For this review, take the finished solid that the model builds, in its own axes (mm). Give positions to 0.01 mm unless a question says otherwise; leave off trailing zeros. Loops run counter-clockwise (first coordinate to the right, second up) from the corner with the lowest first, then second, coordinate; pieces in that order, holes last.
```python
from build123d import *

# Parameters (mm, degrees)
F1_DEPTH        = 6
F2_R            = 1
F3_R            = 5
F4_DEPTH        = 1.8
F6_D            = 2.8
F6_CBORE_D      = 6
F6_CBORE_DEPTH  = 2.5
F7_SIZE         = 3
F9_DEPTH        = 0.4
F10_D           = 2.8
F10_CBORE_D     = 6
F10_CBORE_DEPTH = 2.5
F11_R           = 6.1
F12_DEPTH       = 4
F14_DEPTH       = 1


with BuildPart() as f1:
    # F0 (on Right) → F1 (new body)
    with BuildSketch(Plane.YZ):
        Polygon((40.0512183458, -60), (50, -60), (50, 60), (-50, 60), (-50, -60), (-40, -60), (-29.9487816542, -50), (30.0512183458, -50), align=None)
        with BuildLine():
            Line((2.1213203436, -9.1923881554), (32.9289321881, -40))
            Line((32.9289321881, -40), (-32.9289321881, -40))
            Line((-32.9289321881, -40), (-2.1213203436, -9.1923881554))
            ThreePointArc((-2.1213203436, -9.1923881554), (0, -8.313708499), (2.1213203436, -9.1923881554))
        make_face(mode=Mode.SUBTRACT)
        with BuildLine():
            Line((-9.1923881554, -2.1213203436), (-40, -32.9289321881))
            Line((-40, -32.9289321881), (-40, 32.9289321881))
            Line((-40, 32.9289321881), (-9.1923881554, 2.1213203436))
            ThreePointArc((-9.1923881554, 2.1213203436), (-8.313708499, 0), (-9.1923881554, -2.1213203436))
        make_face(mode=Mode.SUBTRACT)
        with BuildLine():
            Line((40, 32.9289321881), (40, -32.9289321881))
            Line((40, -32.9289321881), (9.1923881554, -2.1213203436))
            ThreePointArc((9.1923881554, -2.1213203436), (8.313708499, 0), (9.1923881554, 2.1213203436))
            Line((9.1923881554, 2.1213203436), (40, 32.9289321881))
        make_face(mode=Mode.SUBTRACT)
        with BuildLine():
            Line((-32.9289321881, 40), (32.9289321881, 40))
            Line((32.9289321881, 40), (2.1213203436, 9.1923881554))
            ThreePointArc((2.1213203436, 9.1923881554), (0, 8.313708499), (-2.1213203436, 9.1923881554))
            Line((-2.1213203436, 9.1923881554), (-32.9289321881, 40))
        make_face(mode=Mode.SUBTRACT)
    extrude(amount=F1_DEPTH)

    # F2
    f2_edges = [f1.edges().sort_by_distance(p)[0] for p in [
        (3, -32.928932, 40),
        (3, 32.928932, 40),
        (3, -40, 32.928932),
        (3, -40, -32.928932),
        (3, -32.928932, -40),
        (3, 40, 32.928932),
        (3, 40, -32.928932),
        (3, 32.928932, -40),
    ]]
    fillet(f2_edges, radius=F2_R)

    # F3 (on face) → F4 (cut)
    with BuildSketch(Plane(origin=(0, 0, 0), x_dir=(0, -1, 0), z_dir=(-1, 0, 0))):
        Circle(F3_R)
    extrude(amount=-F4_DEPTH, mode=Mode.SUBTRACT)

    # F6 (through all)
    with Locations(Plane(origin=(0, 0, 0), x_dir=(0, -1, 0), z_dir=(-1, 0, 0))):
        with Locations((-5, -45), (5, -45)):
            CounterBoreHole(F6_D / 2, F6_CBORE_D / 2, F6_CBORE_DEPTH)

    # F7
    f7_edges = [f1.edges().sort_by_distance(p)[0] for p in [
        (3, -50, 60),
        (3, 50, 60),
        (0, -50, 0),
        (0, 50, 0),
        (0, 0, 60),
    ]]
    chamfer(f7_edges, length=F7_SIZE)

    # F8 (on face) → F9 (join)
    with BuildSketch(Plane(origin=(0, 0, 0), x_dir=(0, -1, 0), z_dir=(-1, 0, 0))):
        with BuildLine():
            Line((-47, 57), (-37, 57))
            ThreePointArc((-37, 57), (-54.0710678119, 64.0710678119), (-47, 47))
            Line((-47, 47), (-47, 57))
        make_face()
        with BuildLine():
            ThreePointArc((47, 47), (54.0710678119, 64.0710678119), (37, 57))
            Line((37, 57), (47, 57))
            Line((47, 57), (47, 47))
        make_face()
        with BuildLine():
            Line((-47, -60), (-47, -50))
            ThreePointArc((-47, -50), (-53.0480452096, -67.9637396456), (-37.3669885172, -57.3157701715))
            Line((-37.3669885172, -57.3157701715), (-40.0512183458, -60))
            Line((-40.0512183458, -60), (-47, -60))
        make_face()
        with BuildLine():
            ThreePointArc((37.3529996858, -57.3664880981), (53.0689735945, -67.9478021811), (47, -50))
            Line((47, -50), (47, -60))
            Line((47, -60), (40, -60))
            Line((40, -60), (37.3529996858, -57.3664880981))
        make_face()
    extrude(amount=-F9_DEPTH)

    # F10 (through all)
    with Locations(Plane(origin=(0, 0, 0), x_dir=(0, 1, 0), z_dir=(-1, 0, 0))):
        with Locations((-4, -50), (45, -50)):
            CounterBoreHole(F10_D / 2, F10_CBORE_D / 2, F10_CBORE_DEPTH)

    # F11 (on face) → F12 (cut)
    with BuildSketch(Plane.YZ.offset(6)):
        with Locations((-40, 50)):
            Circle(F11_R)
    extrude(amount=-F12_DEPTH, mode=Mode.SUBTRACT)

    # F13 (on face) → F14 (join)
    with BuildSketch(Plane.YZ.offset(0.4)):
        with BuildLine():
            Line((47.4, 48.2), (47.4, 47.0080032026))
            Line((47.4, 47.0080032026), (48.3105732452, 48.2))
            Line((48.3105732452, 48.2), (48.3105732452, 51.8))
            Line((48.3105732452, 51.8), (47.4, 53.0080032026))
            Line((47.4, 53.0080032026), (47.4, 51.8))
            ThreePointArc((47.4, 51.8), (47.8460498942, 50.9486832981), (48, 50))
            ThreePointArc((48, 50), (47.8460498942, 49.0513167019), (47.4, 48.2))
        make_face()
    extrude(amount=F14_DEPTH)


solid = f1.part
```
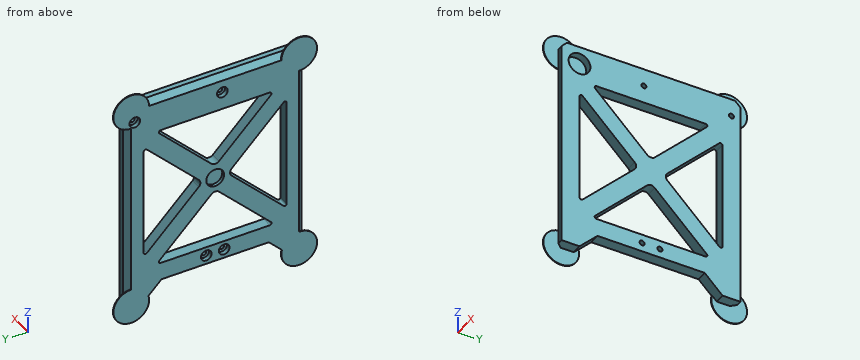
Item 1: Take a section at A-A on y = -19.5. Give the boundary of the cut face in (x, z).
Answer:
outline: (0, -50) - (6, -50) - (6, -40) - (0, -40) - close; (0, -26.57) - (6, -26.57) - (6, -12.43) - (0, -12.43) - close; (0, 12.43) - (6, 12.43) - (6, 26.57) - (0, 26.57) - close; (0, 40) - (6, 40) - (6, 60) - (3, 60) - (0, 57) - close
Item 2: Take a section at B-B on z = 26.5. Give the boundary of the cut face in (x, y).
Answer:
outline: (0, -47) - (3, -50) - (6, -50) - (6, -40) - (0, -40) - close; (0, -33.57) - (6, -33.57) - (6, -19.43) - (0, -19.43) - close; (0, 19.43) - (6, 19.43) - (6, 33.57) - (0, 33.57) - close; (0, 40) - (6, 40) - (6, 50) - (3, 50) - (0, 47) - close
Item 3: For L1, parallel to Z at x = 2, y = -4; L2, parallel to Z at x = 1, y = 25; L3, parallel to Y at x = 4.75, z = 22.5, list the stretches that pass through material, from the lowest coordinate up.
Answer:
L1: z = -50 to -47.83, -42.17 to -40, -11.07 to 11.07, 40 to 47, 53 to 59
L2: z = -50 to -40, -32.07 to -17.93, 17.93 to 32.07, 40 to 58
L3: y = -50 to -40, -29.57 to -15.43, 15.43 to 29.57, 40 to 50
Item 4: Take a section at C-C on x = 4. State how many separate pieces and enclosed holes the cut face has, and give its area (3 significant figures).
Answer:
separate pieces: 1
enclosed holes: 9
area: 6,830 mm2
Item 5: Clearance check with flat-ended pins moving along their axes: pin 1 Ø1.5 at (x, z) = (4, -15.5) entering from -Y; pin 2 Ø3 at (x, z) = (3.5, -5.5) entering from +Y; pin 3 Ø1.7 at (x, y) = (3, 46) entering from -Z; pin 4 Ø2.5 at (y, z) = (-5, -45) entering from +X. State where each tip first meets the part, or that it passes through.
Answer:
pin 1: stops at y = -50
pin 2: stops at y = 50
pin 3: stops at z = -60
pin 4: passes through
